The figure shows three views and two pictorial views of one solid part (mm, origin at its lowest corner). Answer the questions. A direction names the side the tool comes from. Give positions to 0.01 mm unless a question says otherwise; leave off trailing zeros. Write each loop counter-clockwise with the first axis right and the second up, starting at its lowest first coordinate (ties: lowest second). Pieces come first, ordered by that corner, then holes. Notation, with made-up numbers: (-15, 72) - (43, 72) arc R26 cw to (43, 94) - close; hole circle Ø3 at (50, 15.25). An arc over 180 degrees is marked (long way). Answer as CSV lines item,"result". Start each with the question number.
(1) For a pull along Z with two mould halves and no side action, classify the marked faces 3, 4 and 5 as pulls with the +Z half, pulls with the -Z half, needs draft (parallel to the pull), parting line crosses it, or undercut.
(2) Straight lines are drawn through the part: probe 1 along Y at (x, z) = (2.5, 11.5); probe 2 along X at (y, z) = (8, 2.7); probe 3 along Y at (x, z) = (2.5, 5.5). For each, find the intervals that lie inside material, in ascending order.
(3) Find section A-A (z = 8). Write down the section's boundary in (x, y).
(4) Find section C-C (z = 12). State how many separate pieces and enclosed holes the cut face has.
(5) Each of these flat-tipped pins is pushed along its axis until it touches: pin 1 Ø0.9 at (x, y) = (2.5, 8) entering from -Z; pin 2 Ø2.5 at (x, y) = (2.5, 12.5) entering from -Z. Where does it stop, or does it pass through?
(6) For the marked faces 1 and 2, determine the directions among +Z, -Z, +X, -X, +Y, -Y from which every point of the face is accessible in a straight line to the end or side of a thin tool.
(7) Find section B-B (y = 8). Write down the section's boundary in (x, z).
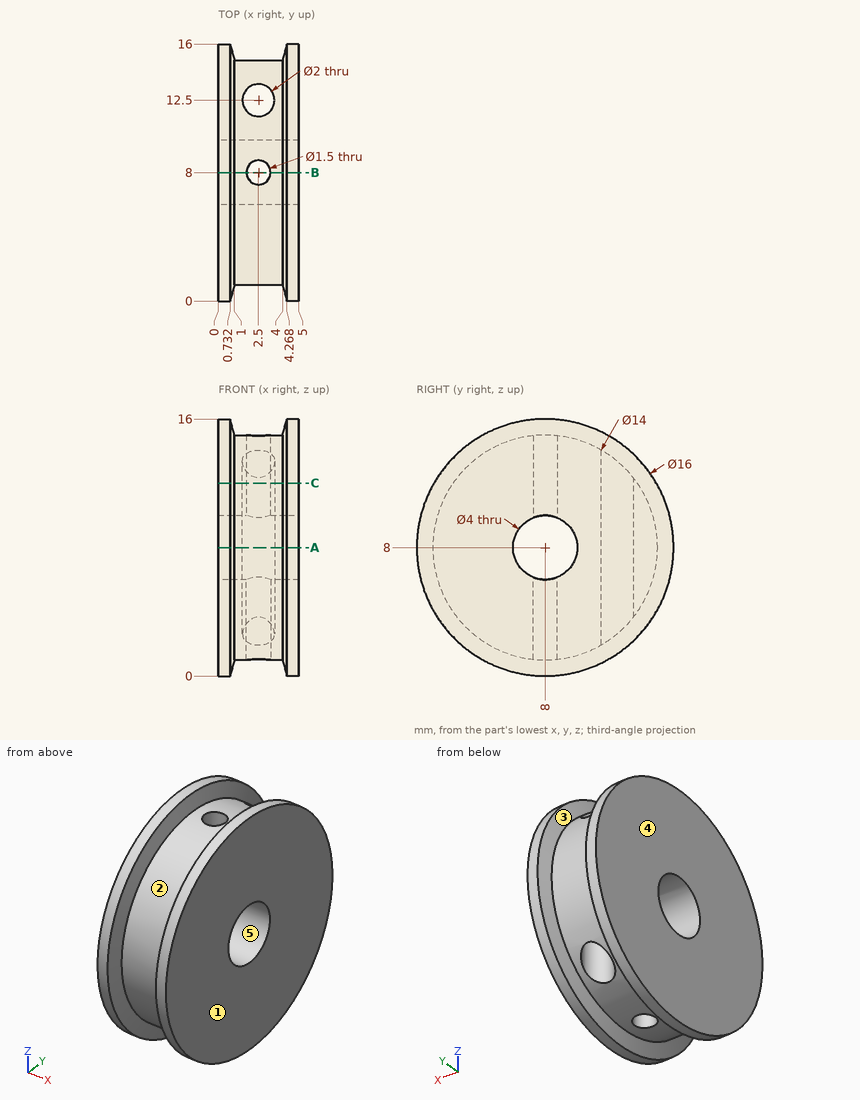
Result set:
1,face 3,"parting line crosses it"
1,face 4,"needs draft"
1,face 5,"undercut"
2,probe 1,"1.94 to 7.25, 8.75 to 11.5, 13.5 to 14.06"
2,probe 2,"0 to 1.75, 3.25 to 5"
2,probe 3,"1.46 to 7.25, 8.75 to 11.5, 13.5 to 14.54"
3,outline,"(0, 0) - (0.73, 0) - (1, 1) - (4, 1) - (4.27, 0) - (5, 0) - (5, 6) - (0, 6) - close; (0, 10) - (5, 10) - (5, 16) - (4.27, 16) - (4, 15) - (1, 15) - (0.73, 16) - (0, 16) - close; hole circle Ø2 at (2.5, 12.5)"
4,separate pieces,"1"
4,enclosed holes,"2"
5,pin 1,"through"
5,pin 2,"z = 1.8"
6,face 1,"+Z, -Z, +X, +Y, -Y"
6,face 2,"none"
7,outline,"(0, 0) - (0.73, 0) - (1, 1) - (1.75, 1) - (1.75, 6) - (0, 6) - close; (0, 10) - (1.75, 10) - (1.75, 15) - (1, 15) - (0.73, 16) - (0, 16) - close; (3.25, 1) - (4, 1) - (4.27, 0) - (5, 0) - (5, 6) - (3.25, 6) - close; (3.25, 10) - (5, 10) - (5, 16) - (4.27, 16) - (4, 15) - (3.25, 15) - close"
